Model file for the job. Use its own axes, mm. Face numbers are marked on the shaded views. Coordinates: 2 decimals unless noted, no trailing zeros. Write each loop counter-clockwise with the first axis right and the second up, starting at its lowest first coordinate (ties: lowest second). Pieces come first, ordered by that corner, then holes. Notation, with made-up numbers: (44.5, 46.5) -> (98.5, 46.5) arc R30 cw to (98.5, 71.5) -> close; hole circle Ø10 at (40.25, 29). An arc over 180 degrees is marked (long way). Answer as a JSON object with one key per item and string values. Group by question number.
from build123d import *

# Parameters (mm, degrees)
SKETCH1_W           = 710
SKETCH1_H           = 494
BOSS_EXTRUDE1_DEPTH = 26
SKETCH2_R           = 3
CUT_EXTRUDE1_DEPTH  = 434.255121147
CUT_EXTRUDE2_REACH  = 435.255
SKETCH3_R           = 2.5
SKETCH4_W           = 40
SKETCH4_H           = 40
BOSS_EXTRUDE2_DEPTH = 570
SKETCH5_W           = 710
SKETCH5_H           = 494
BOSS_EXTRUDE3_DEPTH = 65


with BuildPart() as part:
    # Sketch1 → Boss-Extrude1 (new body)
    with BuildSketch(Plane(origin=(0, 0, 0), x_dir=(1, 0, 0), z_dir=(0, 1, 0))):
        Rectangle(SKETCH1_W, SKETCH1_H)
    extrude(amount=BOSS_EXTRUDE1_DEPTH)

    # Sketch2 → Cut-Extrude1 (cut, through all)
    with BuildSketch(Plane(origin=(0, 26, 0), x_dir=(1, 0, 0), z_dir=(0, 1, 0))):
        with Locations(Location((-67.5, -62, 0), (0, 0, 270))):
            Circle(SKETCH2_R)
        with Locations(Location((-67.5, -197, 0), (0, 0, 270))):
            Circle(SKETCH2_R)
        with Locations(Location((67.5, -197, 0), (0, 0, 270))):
            Circle(SKETCH2_R)
        with Locations(Location((67.5, -62, 0), (0, 0, 270))):
            Circle(SKETCH2_R)
    extrude(amount=-CUT_EXTRUDE1_DEPTH, mode=Mode.SUBTRACT)

    # Sketch3 → Cut-Extrude2 (cut, up to next)
    with BuildSketch(Plane(origin=(0, 26, 0), x_dir=(1, 0, 0), z_dir=(0, 1, 0)), mode=Mode.PRIVATE) as cut_extrude2_sk1:
        with Locations(Location((-335, 121, 0), (0, 0, 270))):
            Circle(SKETCH3_R)
    cut_extrude2_tool1 = extrude(cut_extrude2_sk1.sketch, amount=-CUT_EXTRUDE2_REACH, mode=Mode.PRIVATE) & part.part
    # Sketch3 → Cut-Extrude2 (cut, up to next)
    with BuildSketch(Plane(origin=(0, 26, 0), x_dir=(1, 0, 0), z_dir=(0, 1, 0)), mode=Mode.PRIVATE) as cut_extrude2_sk2:
        with Locations(Location((-335, 86, 0), (0, 0, 270))):
            Circle(SKETCH3_R)
    cut_extrude2_tool2 = extrude(cut_extrude2_sk2.sketch, amount=-CUT_EXTRUDE2_REACH, mode=Mode.PRIVATE) & part.part
    # Sketch3 → Cut-Extrude2 (cut, up to next)
    with BuildSketch(Plane(origin=(0, 26, 0), x_dir=(1, 0, 0), z_dir=(0, 1, 0)), mode=Mode.PRIVATE) as cut_extrude2_sk3:
        with Locations(Location((335, 86, 0), (0, 0, 270))):
            Circle(SKETCH3_R)
    cut_extrude2_tool3 = extrude(cut_extrude2_sk3.sketch, amount=-CUT_EXTRUDE2_REACH, mode=Mode.PRIVATE) & part.part
    # Sketch3 → Cut-Extrude2 (cut, up to next)
    with BuildSketch(Plane(origin=(0, 26, 0), x_dir=(1, 0, 0), z_dir=(0, 1, 0)), mode=Mode.PRIVATE) as cut_extrude2_sk4:
        with Locations(Location((335, 121, 0), (0, 0, 270))):
            Circle(SKETCH3_R)
    cut_extrude2_tool4 = extrude(cut_extrude2_sk4.sketch, amount=-CUT_EXTRUDE2_REACH, mode=Mode.PRIVATE) & part.part
    # Sketch3 → Cut-Extrude2 (cut, up to next)
    with BuildSketch(Plane(origin=(0, 26, 0), x_dir=(1, 0, 0), z_dir=(0, 1, 0)), mode=Mode.PRIVATE) as cut_extrude2_sk5:
        with Locations(Location((335, -85, 0), (0, 0, 270))):
            Circle(SKETCH3_R)
    cut_extrude2_tool5 = extrude(cut_extrude2_sk5.sketch, amount=-CUT_EXTRUDE2_REACH, mode=Mode.PRIVATE) & part.part
    # Sketch3 → Cut-Extrude2 (cut, up to next)
    with BuildSketch(Plane(origin=(0, 26, 0), x_dir=(1, 0, 0), z_dir=(0, 1, 0)), mode=Mode.PRIVATE) as cut_extrude2_sk6:
        with Locations(Location((335, -120, 0), (0, 0, 270))):
            Circle(SKETCH3_R)
    cut_extrude2_tool6 = extrude(cut_extrude2_sk6.sketch, amount=-CUT_EXTRUDE2_REACH, mode=Mode.PRIVATE) & part.part
    # Sketch3 → Cut-Extrude2 (cut, up to next)
    with BuildSketch(Plane(origin=(0, 26, 0), x_dir=(1, 0, 0), z_dir=(0, 1, 0)), mode=Mode.PRIVATE) as cut_extrude2_sk7:
        with Locations(Location((-335, -85, 0), (0, 0, 270))):
            Circle(SKETCH3_R)
    cut_extrude2_tool7 = extrude(cut_extrude2_sk7.sketch, amount=-CUT_EXTRUDE2_REACH, mode=Mode.PRIVATE) & part.part
    # Sketch3 → Cut-Extrude2 (cut, up to next)
    with BuildSketch(Plane(origin=(0, 26, 0), x_dir=(1, 0, 0), z_dir=(0, 1, 0)), mode=Mode.PRIVATE) as cut_extrude2_sk8:
        with Locations(Location((-335, -120, 0), (0, 0, 270))):
            Circle(SKETCH3_R)
    cut_extrude2_tool8 = extrude(cut_extrude2_sk8.sketch, amount=-CUT_EXTRUDE2_REACH, mode=Mode.PRIVATE) & part.part
    add(cut_extrude2_tool1.solids().sort_by_distance((-335, 26, -121))[0], mode=Mode.SUBTRACT)
    add(cut_extrude2_tool2.solids().sort_by_distance((-335, 26, -86))[0], mode=Mode.SUBTRACT)
    add(cut_extrude2_tool3.solids().sort_by_distance((335, 26, -86))[0], mode=Mode.SUBTRACT)
    add(cut_extrude2_tool4.solids().sort_by_distance((335, 26, -121))[0], mode=Mode.SUBTRACT)
    add(cut_extrude2_tool5.solids().sort_by_distance((335, 26, 85))[0], mode=Mode.SUBTRACT)
    add(cut_extrude2_tool6.solids().sort_by_distance((335, 26, 120))[0], mode=Mode.SUBTRACT)
    add(cut_extrude2_tool7.solids().sort_by_distance((-335, 26, 85))[0], mode=Mode.SUBTRACT)
    add(cut_extrude2_tool8.solids().sort_by_distance((-335, 26, 120))[0], mode=Mode.SUBTRACT)

    # Sketch4 → Boss-Extrude2 (add)
    with BuildSketch(Plane.XZ):
        with Locations((-335, 227)):
            Rectangle(SKETCH4_W, SKETCH4_H)
        with Locations((-335, -227)):
            Rectangle(SKETCH4_W, SKETCH4_H)
        with Locations((335, 227)):
            Rectangle(SKETCH4_W, SKETCH4_H)
        with Locations((335, -227)):
            Rectangle(SKETCH4_W, SKETCH4_H)
    extrude(amount=BOSS_EXTRUDE2_DEPTH)

    # Sketch5 → Boss-Extrude3 (add)
    with BuildSketch(Plane.XZ.offset(570)):
        Rectangle(SKETCH5_W, SKETCH5_H)
    extrude(amount=BOSS_EXTRUDE3_DEPTH)


solid = part.part
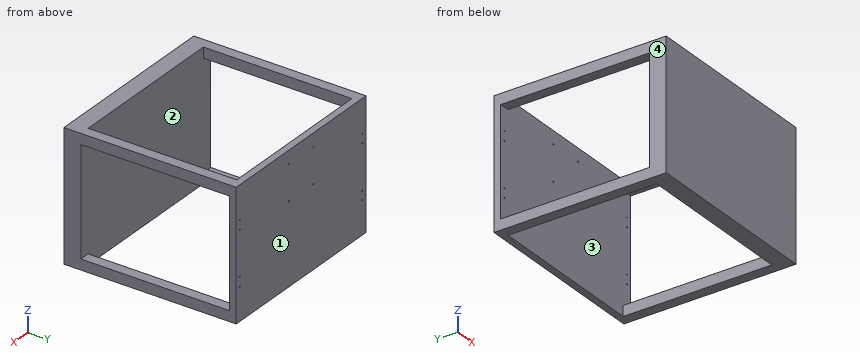
(1) Wall check: probe 1 along Y at (x, z) = (187, -128.5); probe 2 along Z at (x, y) = (-335, 14); probe 3 along X at (y, z) = (10.75, 197). Give the ranges that are in metal, low to high.
(2) Cut at A-A on y = -427.5. List the corners of the cut face in (x, z).
(3) Pin check, flat tips, straight feed: pin 1 (4.5 mm diameter, centred on x = 335, z = 85, fed in from +Y); pin 2 (8 mm diameter, centred on x = 335, z = 120, fed in from +Y). Stop position of each tip, or through.
(4) Cut at B-B on x = -153. List the corners of the cut face in (y, z).
(5) Pull direction Y, two halves, no side cores. Call the marked faces 1, 2, 3 and 4: released by +Y, released by -Y, zero draft, split by the parting line, or undercut.
Results found:
{
 "1": {"probe 1": "y = -635 to -570, 0 to 26", "probe 2": "z = -247 to -123.5, -118.5 to -88.5, -83.5 to 82.5, 87.5 to 117.5, 122.5 to 247", "probe 3": "x = -355 to -70.5, -64.5 to 64.5, 70.5 to 355"},
 "2": {"outline": "(-355, -247) -> (-315, -247) -> (-315, -207) -> (-355, -207) -> close; (-355, 207) -> (-315, 207) -> (-315, 247) -> (-355, 247) -> close; (315, -247) -> (355, -247) -> (355, -207) -> (315, -207) -> close; (315, 207) -> (355, 207) -> (355, 247) -> (315, 247) -> close"},
 "3": {"pin 1": "stops at y = -570", "pin 2": "stops at y = 26"},
 "4": {"outline": "(-635, -247) -> (-570, -247) -> (-570, 247) -> (-635, 247) -> close; (0, -247) -> (26, -247) -> (26, 247) -> (0, 247) -> close"},
 "5": {"face 1": "released by +Y", "face 2": "undercut", "face 3": "undercut", "face 4": "zero draft"}
}
